from build123d import *

# Parameters (mm, degrees)
SKETCH1_W           = 211
SKETCH1_H           = 110
BOSS_EXTRUDE1_DEPTH = 10
SKETCH1_3_W         = 10
SKETCH1_3_H         = 110
BOSS_EXTRUDE2_DEPTH = 14
SKETCH5_W           = 211
SKETCH5_H           = 7.5
CUT_EXTRUDE5_DEPTH  = 3.2
SKETCH6_R           = 3.15
BOSS_EXTRUDE3_DEPTH = 10
CUT_EXTRUDE9_DEPTH  = 2
SKETCH11_W          = 10
SKETCH11_H          = 21.813163886
BOSS_EXTRUDE5_DEPTH = 4
SKETCH12_W          = 10
SKETCH12_H          = 78.75
CUT_EXTRUDE10_DEPTH = 4
CUT_EXTRUDE7_DEPTH  = 3
SKETCH13_W          = 231
SKETCH13_H          = 60.312496228
BOSS_EXTRUDE6_DEPTH = 10


with BuildPart() as part:
    # Sketch1 → Boss-Extrude1 (new body)
    with BuildSketch(Plane(origin=(0, 0, 0), x_dir=(1, 0, 0), z_dir=(0, 1, 0))):
        Rectangle(SKETCH1_W, SKETCH1_H)
    extrude(amount=BOSS_EXTRUDE1_DEPTH)

    # Sketch1_3 → Boss-Extrude2 (add)
    with BuildSketch(Plane(origin=(0, 0, 0), x_dir=(1, 0, 0), z_dir=(0, 1, 0))):
        with Locations((-110.5, 0)):
            Rectangle(SKETCH1_3_W, SKETCH1_3_H)
        with Locations((110.5, 0)):
            Rectangle(SKETCH1_3_W, SKETCH1_3_H)
    extrude(amount=BOSS_EXTRUDE2_DEPTH)

    # Sketch5 → Cut-Extrude5 (cut)
    with BuildSketch(Plane(origin=(0, 10, 0), x_dir=(1, 0, 0), z_dir=(0, 1, 0))):
        Rectangle(SKETCH5_W, SKETCH5_H)
    extrude(amount=-CUT_EXTRUDE5_DEPTH, mode=Mode.SUBTRACT)

    # Sketch6 → Boss-Extrude3 (add)
    with BuildSketch(Plane(origin=(0, 0, 0), x_dir=(1, 0, 0), z_dir=(0, 1, 0))):
        Polygon((-136, 119.243156134), (-106.5, 119.243156134), (104.5, 119.243156134), (135, 119.243156134), (135, 99.243156134), (115.5, 99.243156134), (115.5, 55), (-115.5, 55), (-115.5, 99.243156134), (-136, 99.243156134), align=None)
        with Locations((-127.75, 109)):
            Circle(SKETCH6_R, mode=Mode.SUBTRACT)
        with Locations((127.75, 109)):
            Circle(SKETCH6_R, mode=Mode.SUBTRACT)
        Polygon((-136, -66.252271661), (-115.5, -66.252271661), (-115.5, -55), (-104.100072783, -55), (104.5, -55), (115.5, -55), (115.5, -66.252271661), (136, -66.252271661), (136, -88.065435547), (-136, -88.065435547), align=None)
        with Locations((-127.75, -75.253909377)):
            Circle(SKETCH6_R, mode=Mode.SUBTRACT)
        with Locations((127.75, -75.253909377)):
            Circle(SKETCH6_R, mode=Mode.SUBTRACT)
    extrude(amount=BOSS_EXTRUDE3_DEPTH)

    # Sketch7_2 → Cut-Extrude9 (cut)
    with BuildSketch(Plane.XZ):
        Polygon((-127.75, 69.364936631), (-122.65, 72.309423004), (-122.65, 78.19839575), (-127.75, 81.142882123), (-132.85, 78.19839575), (-132.85, 72.309423004), align=None)
        Polygon((127.75, 69.364936631), (132.85, 72.309423004), (132.85, 78.19839575), (127.75, 81.142882123), (122.65, 78.19839575), (122.65, 72.309423004), align=None)
        Polygon((-127.75, -114.888972746), (-122.65, -111.944486373), (-122.65, -106.055513627), (-127.75, -103.111027254), (-132.85, -106.055513627), (-132.85, -111.944486373), align=None)
        Polygon((127.75, -114.888972746), (132.85, -111.944486373), (132.85, -106.055513627), (127.75, -103.111027254), (122.65, -106.055513627), (122.65, -111.944486373), align=None)
    extrude(amount=-CUT_EXTRUDE9_DEPTH, mode=Mode.SUBTRACT)

    # Sketch11 → Boss-Extrude5 (add)
    with BuildSketch(Plane(origin=(0, 10, 0), x_dir=(1, 0, 0), z_dir=(0, 1, 0))):
        with Locations((-110.5, -77.158853604)):
            Rectangle(SKETCH11_W, SKETCH11_H)
        with Locations((110.5, -77.158853604)):
            Rectangle(SKETCH11_W, SKETCH11_H)
    extrude(amount=BOSS_EXTRUDE5_DEPTH)

    # Sketch12 → Cut-Extrude10 (cut)
    with BuildSketch(Plane(origin=(0, 14, 0), x_dir=(1, 0, 0), z_dir=(0, 1, 0))):
        with Locations((-110.5, -15.625)):
            Rectangle(SKETCH12_W, SKETCH12_H)
        with Locations((110.5, -15.625)):
            Rectangle(SKETCH12_W, SKETCH12_H)
    extrude(amount=-CUT_EXTRUDE10_DEPTH, mode=Mode.SUBTRACT)

    # Sketch7 → Cut-Extrude7 (cut)
    with BuildSketch(Plane.XZ):
        Polygon((-127.75, 69.364936631), (-122.65, 72.309423004), (-122.65, 78.19839575), (-127.75, 81.142882123), (-132.85, 78.19839575), (-132.85, 72.309423004), align=None)
        Polygon((127.75, 69.364936631), (132.85, 72.309423004), (132.85, 78.19839575), (127.75, 81.142882123), (122.65, 78.19839575), (122.65, 72.309423004), align=None)
        Polygon((-127.75, -114.888972746), (-122.65, -111.944486373), (-122.65, -106.055513627), (-127.75, -103.111027254), (-132.85, -106.055513627), (-132.85, -111.944486373), align=None)
        Polygon((127.75, -114.888972746), (132.85, -111.944486373), (132.85, -106.055513627), (127.75, -103.111027254), (122.65, -106.055513627), (122.65, -111.944486373), align=None)
    extrude(amount=-CUT_EXTRUDE7_DEPTH, mode=Mode.SUBTRACT)

    # Sketch13 → Boss-Extrude6 (add)
    with BuildSketch(Plane(origin=(0, 0, 0), x_dir=(1, 0, 0), z_dir=(0, 1, 0))):
        with Locations((0, 149.399404248)):
            Rectangle(SKETCH13_W, SKETCH13_H)
    extrude(amount=BOSS_EXTRUDE6_DEPTH)


solid = part.part
Work out the finished part from the listing and answer in its coordinate system (mm). A direction names the side the tool comes from. Round coordinates to 2 decimals unless told otherwise and drop trailing zeros. Write each loop counter-clockwise with the first axis right and the second up, starting at its lowest first coordinate (ties: lowest second). Pieces come first, ordered by that corner, then holes.
1) A cutting plane is placed at B-B (z = -74.5). Give the vertices of the cut face in (x, y), plus the area to 3 significant figures.
2) A cutting plane is placed at A-A (x = -68.5). Give the vertices of the cut face in (y, z), plus the area to 3 significant figures.
3) Straight lines are drawn through the part: line 1 (X direction, y = 5, z = -109); line 2 (Z direction, x = -127.75, y = 7.5); line 3 (Z direction, x = -15.5, y = 8.75). For each, find the intervals that lie inside material, in ascending order.
4) The mould has two halves that part along X. Classify faces 6 (the flat face through (-136, 5, 77)), 7 (the flat face through (-130, 3, -112)), 8 (the cylindrical face through (-124.745, 6.451, 74.308)), 9 (the flat face through (-111, 14, 77)): pulls with the +X half, pulls with the -X half, needs draft (parallel to the pull), parting line crosses it, or undercut.
5) Given pin 1 Ø3 at (y, z) = (6.5, -138) entering from -X; pin 2 Ø1.2 at (x, y) = (-108.5, 13) entering from -Z; pin 3 Ø5 at (x, y) = (-124.5, 4.5) entering from -Z, each flat-ended and moving along its own axis, determine where each tip first touches the part or whether it passes through.
6) A tool of negligible diameter and unlimited length cuts with its end or side. For faces 1 (the flat face through (-126, 5, 66.252)), 2 (the flat face through (-1, 6.8, 0)), 3 (the flat face through (-124, 10, 77)), 4 (the flat face through (-115.5, 5, -149)), 5 (the flat face through (115.5, 5, -149)), from which of +Z, -Z, +X, -X, +Y, -Y can it reach the whole face along a straight path? Write none if from no direction.
Completed:
1. outline: (-115.5, 0) - (115.5, 0) - (115.5, 10) - (-115.5, 10) - close
1. area: 2,310 mm2
2. outline: (0, -179.56) - (10, -179.56) - (10, -3.75) - (6.8, -3.75) - (6.8, 3.75) - (10, 3.75) - (10, 88.07) - (0, 88.07) - close
2. area: 2,650 mm2
3. line 1: x = -136 to -130.9, -124.6 to 124.6, 130.9 to 135
3. line 2: z = -119.24 to -112.15, -105.85 to -99.24, 66.25 to 72.1, 78.4 to 88.07
3. line 3: z = -179.56 to -3.75, 3.75 to 88.07
4. face 6: pulls with the -X half
4. face 7: undercut
4. face 8: undercut
4. face 9: needs draft
5. pin 1: stops at x = -115.5
5. pin 2: stops at z = -55
5. pin 3: stops at z = -119.24
6. face 1: -X, +Y, -Y
6. face 2: +Y
6. face 3: +Z, -Z, -X, +Y
6. face 4: -Z, -X, +Y, -Y
6. face 5: -Z, +X, +Y, -Y
